For this review, take the finished solid that the model builds, in its own axes (mm). A direction names the side the tool comes from. Coordinates: 2 decimals unless noted, no trailing zeros. Order: outer loops, then holes, each group sorted by start corner. A loop starts at its lowest first (then second) coordinate and runs counter-clockwise, first axis right, second up.
from build123d import *

# Parameters (mm, degrees)
F0_R         = 4.211
F0_W         = 0.5461883944
F0_H         = 48.4801451702
F1_DEPTH     = 25
F2_T1_DEPTH  = 50
F2_T3_DEPTH  = 100
F2_T5_DEPTH  = 67.0975783302
F2_T7_DEPTH  = 67.2386600166
F2_T9_DEPTH  = 67.0975783302
F2_T11_DEPTH = 66.9249549756
F2_T18_ANGLE = 202.5983722588
F2_T20_ANGLE = 202.5983722588
F2_T22_ANGLE = 202.6248548609
F2_T24_ANGLE = 202.6248548609
F2_T26_ANGLE = 201.5951809175
F2_T28_ANGLE = 201.5951809175
F2_T30_ANGLE = 202.6248548609
F2_T32_ANGLE = 202.6248548609


# Not quite as in the source:
# - a fillet or chamfer that OpenCascade refuses, or shapes differently, is made with other operations: its cross-section is extruded or revolved along the edge and cut away or added


with BuildPart() as f1:
    # F0 (on Top) → F1 (new body, symmetric)
    with BuildSketch(Plane.XY):
        with BuildLine():
            Line((7.6582201656, -71.9089287116), (7.6582201656, -23.4287835415))
            ThreePointArc((7.6582201656, -23.4287835415), (17.4241101733, -17.4343516945), (23.4242794808, -7.6719857367))
            Line((23.4242794808, -7.6719857367), (71.7281472729, -7.6719857367))
            Line((71.7281472729, -7.6719857367), (71.7281472729, 8.1906429889))
            Line((71.7281472729, 8.1906429889), (23.2480021027, 8.1906429889))
            ThreePointArc((23.2480021027, 8.1906429889), (17.2293028181, 17.6268930541), (7.6582201656, 23.4287835415))
            Line((7.6582201656, 23.4287835415), (7.6582201656, 71.9089287116))
            Line((7.6582201656, 71.9089287116), (-7.6582201656, 71.9089287116))
            Line((-7.6582201656, 71.9089287116), (-7.6582201656, 23.4287835415))
            ThreePointArc((-7.6582201656, 23.4287835415), (-17.2293028181, 17.6268930541), (-23.2480021027, 8.1906429889))
            Line((-23.2480021027, 8.1906429889), (-71.7281472729, 8.1906429889))
            Line((-71.7281472729, 8.1906429889), (-71.7281472729, -7.6719857367))
            Line((-71.7281472729, -7.6719857367), (-23.4242794808, -7.6719857367))
            ThreePointArc((-23.4242794808, -7.6719857367), (-17.4241101733, -17.4343516945), (-7.6582201656, -23.4287835415))
            Line((-7.6582201656, -23.4287835415), (-7.6582201656, -71.9089287116))
            Line((-7.6582201656, -71.9089287116), (7.6582201656, -71.9089287116))
        make_face()
        Circle(F0_R, mode=Mode.SUBTRACT)
        with Locations((7.9313143628, 47.6688561266)):
            Rectangle(F0_W, F0_H)
    extrude(amount=F1_DEPTH, both=True)

    # F2: fillet of radius 10 on 18 edges, made by hand

    # F2_s2 → F2_t1 (join)
    with BuildSketch(Plane.XY.offset(-25)):
        with BuildLine():
            ThreePointArc((-12.5618550278, 21.2074522892), (-8.9701924441, 24.8597673709), (-7.6582201656, 29.8113503815))
            Line((-7.6582201656, 29.8113503815), (-7.6582201656, 23.4287835415))
            ThreePointArc((-7.6582201656, 23.4287835415), (-10.170862222, 22.4523895387), (-12.5618550278, 21.2074522892))
        make_face()
        with BuildLine():
            ThreePointArc((20.9784825584, 12.9406145096), (24.6161046934, 9.458510237), (29.4894872562, 8.1906429889))
            Line((29.4894872562, 8.1906429889), (23.2480021027, 8.1906429889))
            ThreePointArc((23.2480021027, 8.1906429889), (22.2404146484, 10.6263912316), (20.9784825584, 12.9406145096))
        make_face()
        with BuildLine():
            ThreePointArc((12.5618550278, -21.2074522892), (8.9701924441, -24.8597673709), (7.6582201656, -29.8113503815))
            Line((7.6582201656, -29.8113503815), (7.6582201656, -23.4287835415))
            ThreePointArc((7.6582201656, -23.4287835415), (10.170862222, -22.4523895387), (12.5618550278, -21.2074522892))
        make_face()
        with BuildLine():
            ThreePointArc((-21.2016487218, -12.5716476969), (-24.8536155677, -8.9828148787), (-29.8031922973, -7.6719857367))
            Line((-29.8031922973, -7.6719857367), (-23.4242794808, -7.6719857367))
            ThreePointArc((-23.4242794808, -7.6719857367), (-22.4470496684, -10.1826418734), (-21.2016487218, -12.5716476969))
        make_face()
    extrude(amount=F2_T1_DEPTH)

    # F2_s4 → F2_t3 (cut)
    with BuildSketch(Plane.XY.offset(-50)):
        with BuildLine():
            ThreePointArc((2.3417798344, 71.9089287116), (-4.7292879775, 68.9799965235), (-7.6582201656, 61.9089287116))
            Line((-7.6582201656, 61.9089287116), (-7.6582201656, 71.9089287116))
            Line((-7.6582201656, 71.9089287116), (2.3417798344, 71.9089287116))
        make_face()
        with BuildLine():
            ThreePointArc((71.7281472729, -1.8093570111), (68.7992150847, 5.2617108008), (61.7281472729, 8.1906429889))
            Line((61.7281472729, 8.1906429889), (71.7281472729, 8.1906429889))
            Line((71.7281472729, 8.1906429889), (71.7281472729, -1.8093570111))
        make_face()
        with BuildLine():
            ThreePointArc((-2.3417798344, -71.9089287116), (4.7292879775, -68.9799965235), (7.6582201656, -61.9089287116))
            Line((7.6582201656, -61.9089287116), (7.6582201656, -71.9089287116))
            Line((7.6582201656, -71.9089287116), (-2.3417798344, -71.9089287116))
        make_face()
        with BuildLine():
            ThreePointArc((-71.7281472729, 2.3280142633), (-68.7992150847, -4.7430535485), (-61.7281472729, -7.6719857367))
            Line((-61.7281472729, -7.6719857367), (-71.7281472729, -7.6719857367))
            Line((-71.7281472729, -7.6719857367), (-71.7281472729, 2.3280142633))
        make_face()
    extrude(amount=F2_T3_DEPTH, mode=Mode.SUBTRACT)

    # F2_s6 → F2_t5 (cut)
    with BuildSketch(Plane.XZ.offset(-96.9089287116)):
        with BuildLine():
            ThreePointArc((2.3417798344, -25), (-4.7292879775, -22.0710678119), (-7.6582201656, -15))
            Line((-7.6582201656, -15), (-7.6582201656, -25))
            Line((-7.6582201656, -25), (2.3417798344, -25))
        make_face()
        with BuildLine():
            ThreePointArc((2.3417798344, 25), (-4.7292879775, 22.0710678119), (-7.6582201656, 15))
            Line((-7.6582201656, 15), (-7.6582201656, 25))
            Line((-7.6582201656, 25), (2.3417798344, 25))
        make_face()
    extrude(amount=F2_T5_DEPTH, mode=Mode.SUBTRACT)

    # F2_s8 → F2_t7 (cut)
    with BuildSketch(Plane.YZ.offset(29.4894872562)):
        with BuildLine():
            ThreePointArc((-1.8093570111, -25), (5.2617108008, -22.0710678119), (8.1906429889, -15))
            Line((8.1906429889, -15), (8.1906429889, -25))
            Line((8.1906429889, -25), (-1.8093570111, -25))
        make_face()
        with BuildLine():
            ThreePointArc((-1.8093570111, 25), (5.2617108008, 22.0710678119), (8.1906429889, 15))
            Line((8.1906429889, 15), (8.1906429889, 25))
            Line((8.1906429889, 25), (-1.8093570111, 25))
        make_face()
    extrude(amount=F2_T7_DEPTH, mode=Mode.SUBTRACT)

    # F2_s10 → F2_t9 (cut)
    with BuildSketch(Plane.XZ.offset(29.8113503815)):
        with BuildLine():
            ThreePointArc((-2.3417798344, -25), (4.7292879775, -22.0710678119), (7.6582201656, -15))
            Line((7.6582201656, -15), (7.6582201656, -25))
            Line((7.6582201656, -25), (-2.3417798344, -25))
        make_face()
        with BuildLine():
            ThreePointArc((-2.3417798344, 25), (4.7292879775, 22.0710678119), (7.6582201656, 15))
            Line((7.6582201656, 15), (7.6582201656, 25))
            Line((7.6582201656, 25), (-2.3417798344, 25))
        make_face()
    extrude(amount=F2_T9_DEPTH, mode=Mode.SUBTRACT)

    # F2_s12 → F2_t11 (cut)
    with BuildSketch(Plane.YZ.offset(-96.7281472729)):
        with BuildLine():
            ThreePointArc((2.3280142633, -25), (-4.7430535485, -22.0710678119), (-7.6719857367, -15))
            Line((-7.6719857367, -15), (-7.6719857367, -25))
            Line((-7.6719857367, -25), (2.3280142633, -25))
        make_face()
        with BuildLine():
            ThreePointArc((2.3280142633, 25), (-4.7430535485, 22.0710678119), (-7.6719857367, 15))
            Line((-7.6719857367, 15), (-7.6719857367, 25))
            Line((-7.6719857367, 25), (2.3280142633, 25))
        make_face()
    extrude(amount=F2_T11_DEPTH, mode=Mode.SUBTRACT)

    # F2_s13 → F2_t14 (revolve, cut)
    with BuildSketch(Plane.XZ):
        with BuildLine():
            ThreePointArc((14.211, -25), (7.1399321881, -22.0710678119), (4.211, -15))
            Line((4.211, -15), (4.211, -25))
            Line((4.211, -25), (14.211, -25))
        make_face()
    revolve(axis=Axis((0, 0, -25), (0, 0, 1)), mode=Mode.SUBTRACT)

    # F2_s15 → F2_t16 (revolve, cut)
    with BuildSketch(Plane.XZ):
        with BuildLine():
            ThreePointArc((14.211, 25), (7.1399321881, 22.0710678119), (4.211, 15))
            Line((4.211, 15), (4.211, 25))
            Line((4.211, 25), (14.211, 25))
        make_face()
    revolve(axis=Axis((0, 0, 25), (0, 0, 1)), mode=Mode.SUBTRACT)

    # F2_s17 → F2_t18 (revolve, cut)
    with BuildSketch(Plane(origin=(-19.132963154, 7.963646146, 0), x_dir=(0, 0, 1), z_dir=(-0.9232211344, 0.3842690946, 0))):
        with BuildLine():
            ThreePointArc((25, -47.7675964389), (22.0710678119, -40.696528627), (15, -37.7675964389))
            Line((15, -37.7675964389), (25, -37.7675964389))
            Line((25, -37.7675964389), (25, -47.7675964389))
        make_face()
    revolve(axis=Axis((-29.8031922972, -17.6719857367, 25), (0, 0, 1)), revolution_arc=F2_T18_ANGLE, mode=Mode.SUBTRACT)

    # F2_s19 → F2_t20 (revolve, cut)
    with BuildSketch(Plane(origin=(-19.132963154, 7.963646146, 0), x_dir=(0, 0, 1), z_dir=(-0.9232211344, 0.3842690946, 0))):
        with BuildLine():
            ThreePointArc((-25, -47.7675964389), (-22.0710678119, -40.696528627), (-15, -37.7675964389))
            Line((-15, -37.7675964389), (-25, -37.7675964389))
            Line((-25, -37.7675964389), (-25, -47.7675964389))
        make_face()
    revolve(axis=Axis((-29.8031922972, -17.6719857367, -25), (0, 0, 1)), revolution_arc=F2_T20_ANGLE, mode=Mode.SUBTRACT)

    # F2_s21 → F2_t22 (revolve, cut)
    with BuildSketch(Plane(origin=(-7.9724845558, -19.1292702646, 0), x_dir=(0, 0, 1), z_dir=(-0.3846957743, -0.9230434233, 0))):
        with BuildLine():
            ThreePointArc((25, -47.7676045084), (22.0710678119, -40.6965366966), (15, -37.7676045084))
            Line((15, -37.7676045084), (25, -37.7676045084))
            Line((25, -37.7676045084), (25, -47.7676045084))
        make_face()
    revolve(axis=Axis((17.6582201656, -29.8113503815, 25), (0, 0, 1)), revolution_arc=F2_T22_ANGLE, mode=Mode.SUBTRACT)

    # F2_s23 → F2_t24 (revolve, cut)
    with BuildSketch(Plane(origin=(-7.9724845558, -19.1292702646, 0), x_dir=(0, 0, 1), z_dir=(-0.3846957743, -0.9230434233, 0))):
        with BuildLine():
            ThreePointArc((-25, -47.7676045084), (-22.0710678119, -40.6965366966), (-15, -37.7676045084))
            Line((-15, -37.7676045084), (-25, -37.7676045084))
            Line((-25, -37.7676045084), (-25, -47.7676045084))
        make_face()
    revolve(axis=Axis((17.6582201656, -29.8113503815, -25), (0, 0, 1)), revolution_arc=F2_T24_ANGLE, mode=Mode.SUBTRACT)

    # F2_s25 → F2_t26 (revolve, cut)
    with BuildSketch(Plane(origin=(19.2698363003, -7.6275931455, 0), x_dir=(0, 0, 1), z_dir=(0.9298074451, -0.3680463489, 0))):
        with BuildLine():
            ThreePointArc((25, -47.7672933998), (22.0710678119, -40.6962255879), (15, -37.7672933998))
            Line((15, -37.7672933998), (25, -37.7672933998))
            Line((25, -37.7672933998), (25, -47.7672933998))
        make_face()
    revolve(axis=Axis((29.4894872562, 18.1906429889, 25), (0, 0, 1)), revolution_arc=F2_T26_ANGLE, mode=Mode.SUBTRACT)

    # F2_s27 → F2_t28 (revolve, cut)
    with BuildSketch(Plane(origin=(19.2698363003, -7.6275931455, 0), x_dir=(0, 0, 1), z_dir=(0.9298074451, -0.3680463489, 0))):
        with BuildLine():
            ThreePointArc((-25, -47.7672933998), (-22.0710678119, -40.6962255879), (-15, -37.7672933998))
            Line((-15, -37.7672933998), (-25, -37.7672933998))
            Line((-25, -37.7672933998), (-25, -47.7672933998))
        make_face()
    revolve(axis=Axis((29.4894872562, 18.1906429889, -25), (0, 0, 1)), revolution_arc=F2_T28_ANGLE, mode=Mode.SUBTRACT)

    # F2_s29 → F2_t30 (revolve, cut)
    with BuildSketch(Plane(origin=(7.9724845558, 19.1292702646, 0), x_dir=(0, 0, 1), z_dir=(0.3846957743, 0.9230434233, 0))):
        with BuildLine():
            ThreePointArc((25, -47.7676045084), (22.0710678119, -40.6965366966), (15, -37.7676045084))
            Line((15, -37.7676045084), (25, -37.7676045084))
            Line((25, -37.7676045084), (25, -47.7676045084))
        make_face()
    revolve(axis=Axis((-17.6582201656, 29.8113503815, 25), (0, 0, 1)), revolution_arc=F2_T30_ANGLE, mode=Mode.SUBTRACT)

    # F2_s31 → F2_t32 (revolve, cut)
    with BuildSketch(Plane(origin=(7.9724845558, 19.1292702646, 0), x_dir=(0, 0, 1), z_dir=(0.3846957743, 0.9230434233, 0))):
        with BuildLine():
            ThreePointArc((-25, -47.7676045084), (-22.0710678119, -40.6965366966), (-15, -37.7676045084))
            Line((-15, -37.7676045084), (-25, -37.7676045084))
            Line((-25, -37.7676045084), (-25, -47.7676045084))
        make_face()
    revolve(axis=Axis((-17.6582201656, 29.8113503815, -25), (0, 0, 1)), revolution_arc=F2_T32_ANGLE, mode=Mode.SUBTRACT)


solid = f1.part
1. Machinability: for faces 1 (the face through (-46, -7.672, 0)), 2 (the face through (50.31, 5.18, -22.15)), 3 (the face through (-51.059, -4.665, 22.148)), 4 (the face through (-47, 8.191, 0)), 5 (the face through (-51.059, -4.665, -22.148)), which of the approach directions +Z, -Z, +X, -X, +Y, -Y give a long, thin tool a straight path to every point of the face, cutting with its end or side? Answer none if there is none.
Answer below:
face 1: +Z, -Z, -X, -Y
face 2: -Z, +X, +Y
face 3: +Z, -X, -Y
face 4: +Z, -Z, -X, +Y
face 5: -Z, -X, -Y
2. Take a section at B-B, the plane x = -45. Give the boundary of the cut face in (y, z).
Answer below:
outline: (-7.67, -15) arc R10 ccw to (2.33, -25) - (8.19, -25) - (8.19, 25) - (2.33, 25) arc R10 ccw to (-7.67, 15) - close
3. Take a section at C-C, the plane y = 51. Give the boundary of the cut face in (x, z), plus the area to 3 significant figures.
Answer below:
outline: (-7.66, -15) arc R10 ccw to (2.34, -25) - (8.2, -25) - (8.2, 25) - (2.34, 25) arc R10 ccw to (-7.66, 15) - close
area: 750 mm2
4. Clearance check with flat-ended pins moving along their axes: pin 1 Ø8 at (x, z) = (15.5, 2) entering from +Y; pin 2 Ø1 at (x, z) = (23, 2.5) entering from -Y; pin 3 Ø13.5 at (x, y) = (0, 0) entering from +Z. State where each tip first meets the part, or that it passes through.
Answer below:
pin 1: stops at y = 21.8
pin 2: stops at y = -10.07
pin 3: stops at z = 21.66
5. Take a section at D-D, the plane z = 18.5. Give the boundary of the cut face in (x, y) (1 decimal).
Answer below:
outline: (-71.7, 2.3) arc R10 ccw to (-65.2, -7) - (-29.8, -7) arc R10.6 cw to (-19.5, -15.1) arc R24.6 ccw to (-7.7, -23.4) - (-7.7, -71.9) - (-2.3, -71.9) arc R10 ccw to (7, -65.4) - (7, -29.8) arc R10.6 cw to (15.1, -19.5) arc R24.6 ccw to (23.4, -7.7) - (71.7, -7.7) - (71.7, -1.8) arc R10 ccw to (65.2, 7.6) - (29.5, 7.6) arc R10.6 cw to (19.2, 15.4) arc R24.6 ccw to (7.7, 23.4) - (8.2, 23.4) - (8.2, 71.9) - (2.3, 71.9) arc R10 ccw to (-7, 65.4) - (-7, 29.8) arc R10.6 cw to (-15.1, 19.5) arc R24.6 ccw to (-23.2, 8.2) - (-71.7, 8.2) - close; hole circle Ø9.7 at (0, 0)
6. To check wall thickness, follow L1, parallel to X at y = -60, z = -9; L2, parallel to X at y = 29, z = -16; L3, parallel to Y at x = -30.5, z = -10. State the ranges of each line that lie inside material, in increasing order.
Answer below:
L1: x = -7.66 to 7.66
L2: x = -7.64 to 8.2
L3: y = -7.67 to 8.19
7. Take a section at A-A, the plane z = 8. Give the boundary of the cut face in (x, y), plus the area to 3 significant figures.
Answer below:
outline: (-71.73, 2.33) arc R10 ccw to (-61.73, -7.67) - (-29.8, -7.67) arc R10 cw to (-21.2, -12.57) arc R24.65 ccw to (-7.66, -23.43) - (-7.66, -71.91) - (-2.34, -71.91) arc R10 ccw to (7.66, -61.91) - (7.66, -29.81) arc R10 cw to (12.56, -21.21) arc R24.65 ccw to (23.42, -7.67) - (71.73, -7.67) - (71.73, -1.81) arc R10 ccw to (61.73, 8.19) - (29.49, 8.19) arc R10 cw to (20.98, 12.94) arc R24.65 ccw to (7.66, 23.43) - (8.2, 23.43) - (8.2, 71.91) - (2.34, 71.91) arc R10 ccw to (-7.66, 61.91) - (-7.66, 29.81) arc R10 cw to (-12.56, 21.21) arc R24.65 ccw to (-23.25, 8.19) - (-71.73, 8.19) - close; hole circle Ø8.42 at (0, 0)
area: 4,790 mm2
